The model under review builds one solid part; all positions refer to its coordinate system, in mm. Face numbers are marked on the shaded views. A direction names the side the tool comes from. Give positions to 0.01 mm unless a question says otherwise; leave off trailing zeros. Write each loop counter-clockwise with the first axis right and the second up, starting at its lowest first coordinate (ties: lowest second). Pieces come first, ordered by that corner, then holes. Notation, with made-up numbers: (28, 53.5) -> (61, 53.5) arc R38 cw to (61, 92.5) -> close; hole circle Ø10 at (86, 56.5). An arc over 180 degrees is marked (long way). Use CSV: the item, a comma, the result in double quotes.
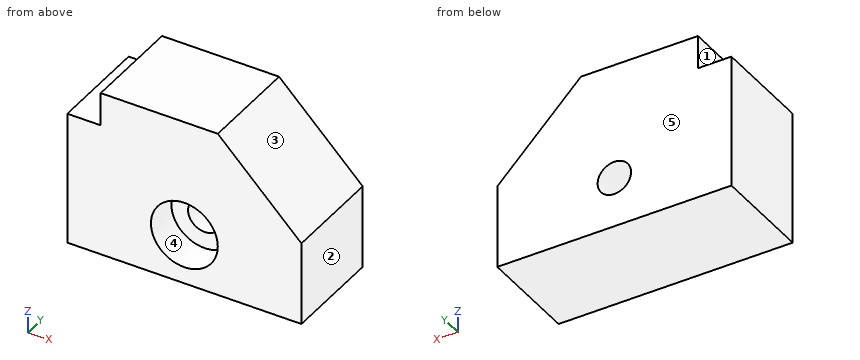
```python
from build123d import *

# Parameters (mm, degrees)
F1_DEPTH = 38.1
F2_R     = 12.7
F3_DEPTH = 12.7
F4_R     = 6.35
F5_DEPTH = 25.401


with BuildPart() as f1:
    # F0 (on Front) → F1 (new body)
    with BuildSketch(Plane.XZ):
        Polygon((0, 50.8), (0, 0), (88.9, 0), (88.9, 31.75), (57.15, 63.5), (12.7, 63.5), (12.7, 50.8), align=None)
    extrude(amount=F1_DEPTH)

    # F2 (on face) → F3 (cut)
    with BuildSketch(Plane.XZ.offset(38.1)):
        with Locations((44.45, 19.05)):
            Circle(F2_R)
    extrude(amount=-F3_DEPTH, mode=Mode.SUBTRACT)

    # F4 (on face) → F5 (cut, through all)
    with BuildSketch(Plane.XZ.offset(25.4)):
        with Locations((44.45, 19.05)):
            Circle(F4_R)
    extrude(amount=-F5_DEPTH, mode=Mode.SUBTRACT)


solid = f1.part
```
Q1. Consider section B-B (y = -27). Write out the cut boundary in (x, z).
Derived:
outline,"(0, 0) -> (88.9, 0) -> (88.9, 31.75) -> (57.15, 63.5) -> (12.7, 63.5) -> (12.7, 50.8) -> (0, 50.8) -> close; hole circle Ø25.4 at (44.45, 19.05)"
Q2. The part is to be moulded in two halves that separate along X. For the marked faces 3, 4 and 5, say which applies: pulls with the +X half, pulls with the -X half, needs draft (parallel to the pull), parting line crosses it, or undercut.
Derived:
face 3,"pulls with the +X half"
face 4,"undercut"
face 5,"needs draft"
Q3. Consider section C-C (z = 19.05). Write out the cut boundary in (x, y).
Derived:
outline,"(0, -38.1) -> (31.75, -38.1) -> (31.75, -25.4) -> (38.1, -25.4) -> (38.1, 0) -> (0, 0) -> close; (50.8, -25.4) -> (57.15, -25.4) -> (57.15, -38.1) -> (88.9, -38.1) -> (88.9, 0) -> (50.8, 0) -> close"
Q4. Consider section D-D (z = 39.5). Write out the cut boundary in (x, y).
Derived:
outline,"(0, -38.1) -> (81.15, -38.1) -> (81.15, 0) -> (0, 0) -> close"
Q5. To check wall thickness, follow probe 1 along Z at (x, y) = (44.45, -13.75); probe 2 along X at (y, z) = (-13, 19); probe 3 along Z at (x, y) = (44.45, -31.5). State the ranges of each line that lie inside material, in increasing order.
Derived:
probe 1,"z = 0 to 12.7, 25.4 to 63.5"
probe 2,"x = 0 to 38.1, 50.8 to 88.9"
probe 3,"z = 0 to 6.35, 31.75 to 63.5"
Q6. Consider section A-A (x = 44.45). Write out the cut boundary in (y, z), then the cut area to 3 significant figures.
Derived:
outline,"(-38.1, 0) -> (0, 0) -> (0, 12.7) -> (-25.4, 12.7) -> (-25.4, 6.35) -> (-38.1, 6.35) -> close; (-38.1, 31.75) -> (-25.4, 31.75) -> (-25.4, 25.4) -> (0, 25.4) -> (0, 63.5) -> (-38.1, 63.5) -> close"
area,"1,770 mm2"
Q7. Insertion check: pin 1 (11.5 mm diameter, centred on x = 44.45, z = 19.05, fed in from +Y); pin 2 (10 mm diameter, centred on y = -12.5, z = 56, fed in from -X); pin 3 (10 mm diameter, centred on x = 5.5, y = -19.5, fed in from +Z). Each pin has a flat end and moves straight along its axis. Give the tip position at first contact, or say it passes through.
Derived:
pin 1,"passes through"
pin 2,"stops at x = 12.7"
pin 3,"stops at z = 50.8"
Q8. Machinability: for the marked faces 1 and 2, which of the approach directions +Z, -Z, +X, -X, +Y, -Y give a long, thin tool a straight path to every point of the face, cutting with its end or side? Answer none if there is none.
Derived:
face 1,"+Z, -X, +Y, -Y"
face 2,"+Z, -Z, +X, +Y, -Y"
